```python
from build123d import *

# Parameters (mm, degrees)
SKETCH_1_R          = 1.7
SKETCH_1_R_2        = 1.8
SKETCH_1_R_3        = 5.7
EXTRUDE_1_DEPTH     = 2.5
SKETCH_2_R          = 10.5
EXTRUDE_2_DEPTH     = 7
SKETCH_4_R          = 1.7
CUT_EXTRUDE_1_DEPTH = 7
CUT_EXTRUDE_2_DEPTH = 3.5
SKETCH_6_R          = 5.7
CUT_EXTRUDE_3_DEPTH = 20


with BuildPart() as part:
    # 草图1 → 凸台-拉伸1 (new body)
    with BuildSketch(Plane(origin=(0, 0, 0), x_dir=(1, 0, 0), z_dir=(0, 1, 0))):
        Polygon((-10, -20), (10, -20), (33.844622395, -43.844622395), (43.844622395, -33.844622395), (20, -10), (20, 20), (-20, 20), (-20, -10), (-43.713203436, -33.713203436), (-33.713203436, -43.713203436), align=None)
        with Locations((-15.5, 15.5)):
            Circle(SKETCH_1_R, mode=Mode.SUBTRACT)
        with Locations((15.5, 15.5)):
            Circle(SKETCH_1_R, mode=Mode.SUBTRACT)
        with Locations((-15.5, -15.5)):
            Circle(SKETCH_1_R_2, mode=Mode.SUBTRACT)
        with Locations((15.5, -15.5)):
            Circle(SKETCH_1_R_2, mode=Mode.SUBTRACT)
        Circle(SKETCH_1_R_3, mode=Mode.SUBTRACT)
        with Locations((-8, 0)):
            Circle(SKETCH_1_R, mode=Mode.SUBTRACT)
        with Locations((0, 8)):
            Circle(SKETCH_1_R, mode=Mode.SUBTRACT)
        with Locations((8, 0)):
            Circle(SKETCH_1_R, mode=Mode.SUBTRACT)
        with Locations((0, -8)):
            Circle(SKETCH_1_R, mode=Mode.SUBTRACT)
        with BuildLine():
            Line((-18.818376618, -21.081118318), (-35.081832586, -37.344574285))
            ThreePointArc((-35.081832586, -37.344574285), (-37.344574285, -37.344574285), (-37.344574285, -35.081832586))
            Line((-37.344574285, -35.081832586), (-21.081118318, -18.818376618))
            ThreePointArc((-21.081118318, -18.818376618), (-18.818376618, -18.818376618), (-18.818376618, -21.081118318))
        make_face(mode=Mode.SUBTRACT)
        with BuildLine():
            Line((21.081118316, -18.818376616), (37.344574284, -35.081832584))
            ThreePointArc((37.344574284, -35.081832584), (37.344574284, -37.344574284), (35.081832584, -37.344574284))
            Line((35.081832584, -37.344574284), (18.818376616, -21.081118316))
            ThreePointArc((18.818376616, -21.081118316), (18.818376616, -18.818376616), (21.081118316, -18.818376616))
        make_face(mode=Mode.SUBTRACT)
    extrude(amount=EXTRUDE_1_DEPTH)

    # 草图2 → 凸台-拉伸2 (add)
    with BuildSketch(Plane(origin=(0, 2.5, 0), x_dir=(1, 0, 0), z_dir=(0, 1, 0))):
        Circle(SKETCH_2_R)
    extrude(amount=EXTRUDE_2_DEPTH)

    # 草图4 → 切除-拉伸1 (cut)
    with BuildSketch(Plane.XZ.offset(-2.5)):
        with Locations((0, -8)):
            Circle(SKETCH_4_R)
        with Locations((-8, 0)):
            Circle(SKETCH_4_R)
        with Locations((8, 0)):
            Circle(SKETCH_4_R)
        with Locations((0, 8)):
            Circle(SKETCH_4_R)
    extrude(amount=-CUT_EXTRUDE_1_DEPTH, mode=Mode.SUBTRACT)

    # 草图5 → 切除-拉伸2 (cut)
    with BuildSketch(Plane(origin=(0, 2.5, 0), x_dir=(1, 0, 0), z_dir=(0, 1, 0))):
        Polygon((-4.766838493, 0), (-6.383419246, 2.8), (-11.233161507, 2.8), (-11.233161507, -2.8), (-6.383419246, -2.8), align=None)
        Polygon((4.766838493, 0), (6.383419246, -2.8), (11.233161507, -2.8), (11.233161507, 2.8), (6.383419246, 2.8), align=None)
        Polygon((-2.8, 11.233161507), (-2.8, 6.383419246), (0, 4.766838493), (2.8, 6.383419246), (2.8, 11.233161507), align=None)
        Polygon((0, -4.766838493), (-2.8, -6.383419246), (-2.8, -11.233161507), (2.8, -11.233161507), (2.8, -6.383419246), align=None)
    extrude(amount=CUT_EXTRUDE_2_DEPTH, mode=Mode.SUBTRACT)

    # 草图6 → 切除-拉伸3 (cut)
    with BuildSketch(Plane.XZ.offset(-2.5)):
        Circle(SKETCH_6_R)
    extrude(amount=-CUT_EXTRUDE_3_DEPTH, mode=Mode.SUBTRACT)


solid = part.part
```
Can you work these out from the model? Positions are in its coordinate system, mm. A direction names the side the tool comes from. Round coordinates to 2 decimals unless told otherwise and drop trailing zeros. Loops run counter-clockwise (first coordinate to the right, second up) from the corner with the lowest first, then second, coordinate; pieces in that order, holes last. Notation, with made-up numbers: (-9, 73) -> (11, 73) arc R26 cw to (11, 93) -> close; hole circle Ø10 at (-1.75, 83). An arc over 180 degrees is marked (long way). One line per item, written item: value. Start each with the question number.
1. If I drill on probe 1 along X at (y, z) = (0.55, 0); probe 2 along X at (y, z) = (0.85, -8), over which ranges is the centre line in solid material (lowest first)?
2. If we section it at D-D, the plane z = 15.5: Write out the boundary of the cut face in (x, y), then the cut area to 4 significant figures.
3. If we section it at A-A, the plane z = 0: Give the number of separate pieces and of enclosed holes in the cut face, then the cut area to 3 significant figures.
4. If we section it at C-C, the plane y = 5: Write out the boundary of the cut face in (x, z).
5. For faces 1 (the flat face through (2.8, 4, -8)), 2 (the flat face through (20, 1, -5)), 3 (the flat face through (-1, 6, 10)), 4 (the flat face through (-10, 6, 0)), 5 (the flat face through (22, 1, 32)), which set-ups out of +Z, -Z, +X, -X, +Y, -Y let a thin tool reach every point of the face, with its end or its side?
6. If we mould it in two halves opening along X, with no side actions, what happens to faces 6 (the flat face through (-20, 1, -5)), 7 (the flat face through (-22, 1, 32)), 8 (the cylindrical face through (-37.32, 1.23, 37.37)), 9 (the cylindrical face through (10, 6, -3.2))? For each: pulls with the +X half, pulls with the -X half, needs draft (parallel to the pull), parting line crosses it, or undercut.
7. For pin 1 (2.5 mm diameter, centred on x = 8, z = 0, fed in from -Y); pin 2 (2 mm diameter, centred on y = 1, z = -7.5, fed in from -X); pin 3 (1.8 mm diameter, centred on y = 4.5, z = 8, fed in from -X); pin 4 (1 mm diameter, centred on x = 8.5, y = 3.5, fed in from +Z), each with a flat end and sliding along its axis, tell me the tip position at first contact or that it passes through.
Calculated:
1. probe 1: x = -20 to -9.7, -6.3 to -5.7, 5.7 to 6.3, 9.7 to 20
1. probe 2: x = -20 to -1.7, 1.7 to 20
2. outline: (-25.5, 0) -> (-17.3, 0) -> (-17.3, 2.5) -> (-25.5, 2.5) -> close; (-13.7, 0) -> (13.7, 0) -> (13.7, 2.5) -> (-13.7, 2.5) -> close; (17.3, 0) -> (25.5, 0) -> (25.5, 2.5) -> (17.3, 2.5) -> close
2. area: 109.5 mm²
3. separate pieces: 8
3. enclosed holes: 0
3. area: 64.3 mm²
4. outline: (-10.12, -2.8) arc R10.5 ccw to (-2.8, -10.12) -> (-2.8, -6.38) -> (-1.34, -5.54) arc R5.7 cw to (-5.54, -1.34) -> (-6.38, -2.8) -> close; (-10.12, 2.8) -> (-6.38, 2.8) -> (-5.54, 1.34) arc R5.7 cw to (-1.34, 5.54) -> (-2.8, 6.38) -> (-2.8, 10.12) arc R10.5 ccw to start; (1.34, -5.54) -> (2.8, -6.38) -> (2.8, -10.12) arc R10.5 ccw to (10.12, -2.8) -> (6.38, -2.8) -> (5.54, -1.34) arc R5.7 cw to start; (1.34, 5.54) arc R5.7 cw to (5.54, 1.34) -> (6.38, 2.8) -> (10.12, 2.8) arc R10.5 ccw to (2.8, 10.12) -> (2.8, 6.38) -> close
5. face 1: -Z
5. face 2: -Z, +X, +Y, -Y
5. face 3: +Z
5. face 4: -X
5. face 5: +Z, +Y, -Y
6. face 6: pulls with the -X half
6. face 7: undercut
6. face 8: undercut
6. face 9: parting line crosses it
7. pin 1: passes through
7. pin 2: stops at x = -20
7. pin 3: stops at x = -7.74
7. pin 4: stops at z = 6.8
